Geometry: final body of the model. Coordinates: model frame, mm. A direction names the side the tool comes from. Round coordinates to 2 decimals unless told otherwise and drop trailing zeros. Loops run counter-clockwise (first coordinate to the right, second up) from the corner with the lowest first, then second, coordinate; pieces in that order, holes last. Notation, with made-up numbers: (24, -23) -> (38, -23) arc R18 cw to (38, 12) -> close; hole circle Ø4 at (-31.5, 59). An arc over 180 degrees is marked (long way). Answer in a Markdown table with one row per item.
```python
from build123d import *

# Parameters (mm, degrees)
BOSS_EXTRUDE1_DEPTH = 2.9


with BuildPart() as part:
    # Sketch2 → Boss-Extrude1 (new body)
    with BuildSketch(Plane.XY):
        Polygon((6.527918297, 15.78), (3.130322537, 3.1), (20.869677463, 3.1), (17.472081703, 15.78), (27, 15.78), (27, 18.78), (-3, 18.78), (-3, 15.78), align=None)
    extrude(amount=-BOSS_EXTRUDE1_DEPTH)

    # Fillet1
    # a fillet whose section is not a circle: 0.3 mm, written as the material it takes off along each edge
    with BuildSketch(Plane(origin=(3.130322537, 3.1, 0.97741903), x_dir=(0.2588190451025178, 0.9659258262890691, 0), z_dir=(0, 0, -1)), Plane(origin=(20.869677463, 3.1, 0.97741903), x_dir=(-1, 0, 0), z_dir=(0, 0, -1))) as fillet1_piece_1:
        with BuildLine():
            add(Edge.make_bspline([(0.390967612, 0), (0.328357725, 0), (0.265747838, 0), (0.130034743, 0.031807338), (0.064378997, 0.117371571), (0.068780602, 0.2566927), (0.084985233, 0.317169207), (0.101189864, 0.377645714)], knots=[0, 0, 0, 0, 0, 0, 0.5, 0.5, 1, 1, 1, 1, 1, 1], degree=5))
            Line((0.101189864, 0.377645714), (0, 0))
            Line((0, 0), (0.390967612, 0))
        make_face()
    extrude(amount=4.854838059, mode=Mode.SUBTRACT)

    # Fillet2
    # a fillet whose section is not a circle: 0.2 mm, written as the material it adds along each edge
    with BuildSketch(Plane(origin=(6.527918297, 15.78, 0), x_dir=(-0.25881904510252, -0.9659258262890685, 0), z_dir=(0, 0, -1)), Plane(origin=(17.472081703, 15.78, 0), x_dir=(1, 0, 0), z_dir=(0, 0, -1))) as fillet2_piece_1:
        with BuildLine():
            add(Edge.make_bspline([(0.260645075, 0), (0.21890515, 0), (0.177165225, 0), (0.086689828, 0.021204892), (0.042919331, 0.078247714), (0.045853734, 0.171128466), (0.056656822, 0.211446138), (0.067459909, 0.251763809)], knots=[0, 0, 0, 0, 0, 0, 0.5, 0.5, 1, 1, 1, 1, 1, 1], degree=5))
            Line((0.067459909, 0.251763809), (0, 0))
            Line((0, 0), (0.260645075, 0))
        make_face()
    extrude(amount=2.9)


solid = part.part
```
Item 1: Ray query, L1, parallel to X at y = 15.5, z = -1.3; L2, parallel to Y at x = 22, z = -2.15; L3, parallel to X at y = 14.75, z = -0.55. Return the intervals inside material, ascending.
Ans:
| item | result |
|---|---|
| L1 | 6.45 to 17.55 |
| L2 | 15.78 to 18.78 |
| L3 | 6.25 to 17.75 |
Item 2: First-contact query: P1, Ø0.9, axis at x = 21.5, z = -1.5, coming from the -Y side. Flat tip, straight axial feed; report the tip coordinate or a pass-through.
Ans:
| item | result |
|---|---|
| P1 | y = 15.78 |
Item 3: Set-up query: faces 4 (the flat face through (2, 15.78, -1)), 5 (the flat face through (19.177, 9.418, -1.43)), 6 (the flat face through (10, 12, -2.9)). Return all of +Z, -Z, +X, -X, +Y, -Y with unobstructed straight access to the full face (end or side cutting, diameter ignored); none if empty.
Ans:
| item | result |
|---|---|
| face 4 | +Z, -Z, -X |
| face 5 | +Z, -Z, +X |
| face 6 | -Z, +X, -X, +Y, -Y |
Item 4: Section query B-B, the plane y = 13. Output: boundary loops of the cut face in (x, z).
Ans:
| item | result |
|---|---|
| outline | (5.78, -2.9) -> (18.22, -2.9) -> (18.22, 0) -> (5.78, 0) -> close |
Item 5: Mould query, pull axis Y, two halves, no side actions, for faces 1 (the flat face through (22, 15.78, -1)), 2 (the flat face through (27, 17, -1)), 3 (the flat face through (12, 3.1, -1)). Classes: released by +Y, released by -Y, zero draft, split by the parting line, or undercut.
Ans:
| item | result |
|---|---|
| face 1 | undercut |
| face 2 | zero draft |
| face 3 | released by -Y |
Item 6: Section query A-A, the plane x = 24. Output: boundary loops of the cut face in (y, z).
Ans:
| item | result |
|---|---|
| outline | (15.78, -2.9) -> (18.78, -2.9) -> (18.78, 0) -> (15.78, 0) -> close |
